Verification items for the finished model (mm, model axes). Face numbers are marked on the shaded views. A direction names the side the tool comes from. Coordinates: 2 decimals unless noted, no trailing zeros. Order: outer loops, then holes, each group sorted by start corner. A loop starts at its lowest first (then second) coordinate and runs counter-clockwise, first axis right, second up. Notation, with made-up numbers: M 78,69 L 102,69 A14 cw 102,84 Z; hole C 67,-32.75 d9. An arc over 180 degrees is marked long. Use one line per item in the form item = value. Start each with the question number.
Solid Edge part; units mm, degrees
sketch "Sketch1" plane through (0, 0, 0) normal (0, 0, 1) x (1, 0, 0)
  circle A0 centre (0, 0) radius 2.5
extrude "Protrusion1" add sketch "Sketch1" along normal blind 24
sketch "Sketch2" plane through (0, 0, 24) normal (0, 0, 1) x (1, 0, 0)
  circle A0 centre (0, 0) radius 11
extrude "ExtrudedProtrusion_2" add sketch "Sketch2" against normal blind 2
sketch "Sketch3" plane through (0, 0, 24) normal (0, 0, 1) x (1, 0, 0)
  line L0 (-15.6, -17.6) -> (15.6, -17.6)
  line L1 (15.6, -17.6) -> (17.6, -15.6)
  line L2 (17.6, -15.6) -> (17.6, 15.6)
  line L3 (15.6, 17.6) -> (17.6, 15.6)
  line L4 (15.6, 17.6) -> (-15.6, 17.6)
  line L5 (-15.6, 17.6) -> (-17.6, 15.6)
  line L6 (-17.6, 15.6) -> (-17.6, -15.6)
  line L7 (-15.6, -17.6) -> (-17.6, -15.6)
extrude "ExtrudedProtrusion_3" add sketch "Sketch3" along normal blind 36
hole "Hole_1" at (-13, -13, 24) direction (0, 0, 1) diameter 2.459 depth 2.5 thread major 3 thread length 2.5
hole "Hole1" at (-13, 13, 24) direction (0, 0, 1) diameter 2.459 depth 2.5 thread major 3 thread length 2.5
hole "Hole2" at (13, 13, 24) direction (0, 0, 1) diameter 2.459 depth 2.5 thread major 3 thread length 2.5
hole "Hole3" at (13, -13, 24) direction (0, 0, 1) diameter 2.459 depth 2.5 thread major 3 thread length 2.5
extrude "ExtrudedProtrusion_4" [suppressed]
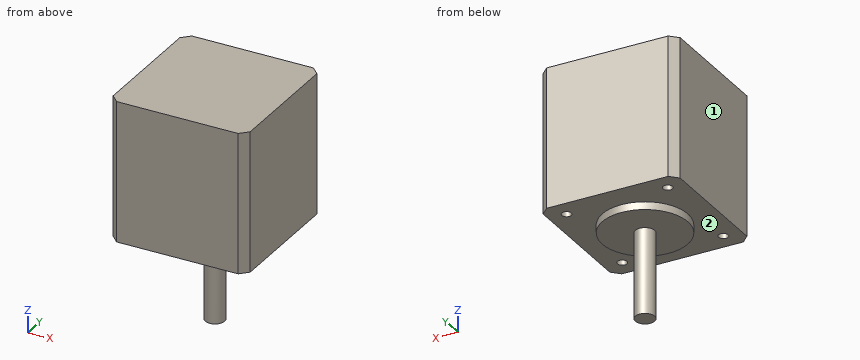
1. Material ranges on line 1 along Y through (x, z) = (-13, 25); line 2 along Z through (x, y) = (16, -5), recorded low to high.
2. Cross-section at C-C on z = 17.5. Enter the section's corners in (x, y), and give its area (3 significant figures).
3. Cross-section at A-A on y = 0. Enter the section's corners in (x, z).
4. Cross-section at D-D on x = 7.5. Enter the section's corners in (y, z), and give its area (3 significant figures).
5. Depth check by flat-ended pin: P1, Ø1.2, axis at x = 13, y = 13, coming from the -Z side; P2, Ø3, axis at y = -1, z = 15, coming from the -X side; P3, Ø8, axis at x = 14, y = -11.5, coming from the -Z side; P4, Ø6, axis at x = -6.5, z = 6.5, coming from the +Y side. Enter the tip coordinate at first touch or a pass-through.
6. Tool access check on the marked faces 1 and 2. Record the directions out of +Z, -Z, +X, -X, +Y, -Y that give a thin tool (end or side, any length) a straight path to the whole face; none if there is none.
Final values:
q1.line_1 = -17.6 to -14.23, -11.77 to 11.77, 14.23 to 17.6
q1.line_2 = 24 to 60
q2.outline = C 0,0 d5
q2.area = 19.6 mm2
q3.outline = M -17.6,24 L -11,24 L -11,22 L -2.5,22 L -2.5,0 L 2.5,0 L 2.5,22 L 11,22 L 11,24 L 17.6,24 L 17.6,60 L -17.6,60 Z
q4.outline = M -17.6,24 L -8.05,24 L -8.05,22 L 8.05,22 L 8.05,24 L 17.6,24 L 17.6,60 L -17.6,60 Z
q4.area = 1,300 mm2
q5.P1 = 26.5
q5.P2 = -2.5
q5.P3 = 24
q5.P4 = through
q6.face_1 = +Z, -Z, -X, +Y, -Y
q6.face_2 = -Z
